Could you check a few things on this model? Use its own coordinates, in mm. A direction names the side the tool comes from. Give positions to 0.01 mm unless a question says otherwise; leave off trailing zeros. Loops run counter-clockwise (first coordinate to the right, second up) from the corner with the lowest first, then second, coordinate; pieces in that order, holes last. Notation, with made-up numbers: (83, 84) - (107, 84) arc R17 cw to (107, 101) - close; hole circle Ø8 at (3, -32). An arc over 180 degrees is marked (long way). Write each question's results on one line, items separated by ' | '. Start each with the question number.
(1) For pin 1 (2.5 mm diameter, centred on y = 28, z = 16.5, fed in from +X); pin 2 (2.5 mm diameter, centred on x = -2, z = 7, fed in from -Y); pin 3 (2 mm diameter, centred on x = -20.5, z = 11, fed in from +Y), each with a flat end and sliding along its axis, tell me the tip position at first contact or that it passes through.
(2) Suppose I cut it at C-C (z = 7.75). Please give me the cut outline in (x, y), and give its area (3 significant figures).
(3) I need wall thicknesses on line 1 (X direction, y = 35, z = 16); line 2 (Y direction, x = 0, z = 15.9); line 3 (Y direction, x = 0, z = 4.65). Which ranges of each line are inside material? Lowest first, please.
(4) Suppose I cut it at B-B (x = -10). Please give me the cut outline in (y, z).
(5) Suppose I cut it at D-D (x = 14.5). Please give me the cut outline in (y, z).
(6) If we mould it in two halves opening along X, with no side actions, what happens to faces 5 (the face through (8.894, 43.96, 10.902)), 6 (the face through (22.88, 44.49, 11.1)), 7 (the face through (0, 41, 18))? For each: released by +X, released by -X, zero draft, split by the parting line, or undercut.
(7) On a 3-axis mill with a long thin cutter (end or side, diameter ignored), from which of +Z, -Z, +X, -X, +Y, -Y can I reach the whole of each face in a straight line? I mean faces 1 (the face through (0.46, 28.84, 4.49)), 2 (the face through (-19, 31, 16)), 3 (the face through (2.211, 32.947, 16.479)), 4 (the face through (6, 22, 9)). Say none if no direction works.
(8) Suppose I cut it at A-A (x = 0). Please give me the cut outline in (y, z), and give its area (3 significant figures).
from build123d import *
from build123d.topology import SkipClean

# Parameters (mm, degrees)
CROQUIS3_W                   = 38
CROQUIS3_H                   = 38
SALIENTE_EXTRUIR9_DEPTH      = 1
SALIENTE_EXTRUIR10_START     = -11
SALIENTE_EXTRUIR10_OUTLINE_W = 38
SALIENTE_EXTRUIR10_OUTLINE_H = 38
SALIENTE_EXTRUIR10_DEPTH     = 10
CROQUIS13_W                  = 38
CROQUIS13_H                  = 38
SALIENTE_EXTRUIR15_DEPTH     = 3
CROQUIS14_R                  = 1.5
CORTAR_EXTRUIR1_DEPTH        = 14
CROQUIS15_W                  = 38
CROQUIS15_H                  = 24.129942315
CROQUIS15_R                  = 1.5
CROQUIS15_R_2                = 3.5
SALIENTE_EXTRUIR16_DEPTH     = 1
CORTAR_EXTRUIR2_DEPTH        = 14
CROQUIS17_R                  = 1.5
SALIENTE_EXTRUIR17_DEPTH     = 5
CROQUIS18_R                  = 1.5
CROQUIS18_W                  = 12
CROQUIS18_H                  = 12
SALIENTE_EXTRUIR18_DEPTH     = 5
CORTAR_EXTRUIR3_DEPTH        = 3
CROQUIS20_R                  = 3
CROQUIS20_R_2                = 1.5
SALIENTE_EXTRUIR19_DEPTH     = 3
REDONDEO11_R                 = 1


# Read off the part's stored shape, not the designer's step: Saliente-Extruir10
with BuildPart() as part:
    # Croquis3 → Saliente-Extruir9 (new body)
    with BuildSketch(Plane.XY.offset(5)):
        Polygon((19, -5.370057685), (26.870057685, 2.5), (26.870057685, 40.5), (19, 48.370057685), (-19, 48.370057685), (-26.870057685, 40.5), (-26.870057685, 2.5), (-19, -5.370057685), align=None)
        with Locations((0, 21.5)):
            Rectangle(CROQUIS3_W, CROQUIS3_H, mode=Mode.SUBTRACT)
    extrude(amount=-SALIENTE_EXTRUIR9_DEPTH)

    # Saliente-Extruir10 outline → Saliente-Extruir10 (add)
    with BuildSketch(Plane(origin=(0, 0, 4), x_dir=(-1, 0, 0), z_dir=(0, 0, -1)).offset(SALIENTE_EXTRUIR10_START)):
        Polygon((-26.870057685, 2.5), (-19, -5.370057685), (19, -5.370057685), (26.870057685, 2.5), (26.870057685, 40.5), (19, 48.370057685), (-19, 48.370057685), (-26.870057685, 40.5), align=None)
        with Locations((0, 21.5)):
            Rectangle(SALIENTE_EXTRUIR10_OUTLINE_W, SALIENTE_EXTRUIR10_OUTLINE_H, mode=Mode.SUBTRACT)
    extrude(amount=SALIENTE_EXTRUIR10_DEPTH)

    # Croquis13 → Saliente-Extruir15 (add)
    with BuildSketch(Plane.XY.offset(15)):
        with BuildLine():
            Line((-22.5, 44.870057685), (-22.5, -1))
            Line((-22.5, -1), (22.5, -1))
            Line((22.5, -1), (22.5, 44.870057685))
            Line((22.5, 44.870057685), (19.292893219, 48.077164466))
            ThreePointArc((19.292893219, 48.077164466), (18.96846987, 48.293937218), (18.585786438, 48.370057685))
            Line((18.585786438, 48.370057685), (-18.585786438, 48.370057685))
            ThreePointArc((-18.585786438, 48.370057685), (-18.96846987, 48.293937218), (-19.292893219, 48.077164466))
            Line((-19.292893219, 48.077164466), (-22.5, 44.870057685))
        make_face()
        with Locations((0, 21.5)):
            Rectangle(CROQUIS13_W, CROQUIS13_H, mode=Mode.SUBTRACT)
    extrude(amount=SALIENTE_EXTRUIR15_DEPTH)

    # Croquis14 → Cortar-Extruir1 (cut)
    with BuildSketch(Plane(origin=(0, 0, 4), x_dir=(-1, 0, 0), z_dir=(0, 0, -1))):
        with Locations((10, 44.97415474)):
            Circle(CROQUIS14_R)
        with Locations(Location((-10, 44.97415474, 0), (0, 0, 180))):
            Circle(CROQUIS14_R)
    extrude(amount=-CORTAR_EXTRUIR1_DEPTH, mode=Mode.SUBTRACT)

    # Croquis15 → Saliente-Extruir16 (add)
    with BuildSketch(Plane(origin=(0, 0, 4), x_dir=(-1, 0, 0), z_dir=(0, 0, -1))):
        with Locations((0, 28.435028843)):
            Rectangle(CROQUIS15_W, CROQUIS15_H)
        with Locations((0, 34.97415474)):
            Circle(CROQUIS15_R, mode=Mode.SUBTRACT)
        with Locations((0, 25.370057685)):
            Circle(CROQUIS15_R_2, mode=Mode.SUBTRACT)
    extrude(amount=-SALIENTE_EXTRUIR16_DEPTH)

    # Croquis16 → Cortar-Extruir2 (cut)
    with BuildSketch(Plane(origin=(0, 0, 4), x_dir=(-1, 0, 0), z_dir=(0, 0, -1))):
        Polygon((-19, 2.5), (-19, 16.370057685), (-26.870057685, 24.24011537), (-26.870057685, 2.5), (-19, -5.370057685), (19, -5.370057685), (26.870057685, 2.5), (26.870057685, 24.24011537), (19, 16.370057685), (19, 2.5), align=None)
    extrude(amount=-CORTAR_EXTRUIR2_DEPTH, mode=Mode.SUBTRACT)

    # Croquis17 → Saliente-Extruir17 (add)
    with SkipClean():  # the faces are left unmerged after this step: merging them gives an invalid solid
        with BuildSketch(Plane.XY.offset(5)):
            Polygon((6, 31.370057685), (6, 25.370057685), (6, 19.370057685), (6, 16.370057685), (19, 16.370057685), (19, 40.5), (-19, 40.5), (-19, 16.370057685), (-6, 16.370057685), (-6, 19.370057685), (-6, 31.370057685), align=None)
            with Locations((0, 34.97415474)):
                Circle(CROQUIS17_R, mode=Mode.SUBTRACT)
        extrude(amount=SALIENTE_EXTRUIR17_DEPTH)
    add(part.part.scale(1), mode=Mode.REPLACE)  # the faces are merged on a copy

    # Croquis18 → Saliente-Extruir18 (add)
    # profile 1 of 2: a face of its own
    with BuildSketch(Plane.XY.offset(10)):
        Polygon((-6, 31.370057685), (6, 31.370057685), (6, 16.370057685), (19, 16.370057685), (19, 40.5), (-19, 40.5), (-19, 16.370057685), (-6, 16.370057685), align=None)
        with Locations(Location((0, 34.97415474, 0), (0, 0, 180))):
            Circle(CROQUIS18_R, mode=Mode.SUBTRACT)
    # profile 2 of 2: a face of its own
    with BuildSketch(Plane.XY.offset(10)):
        with Locations((0, 25.370057685)):
            Rectangle(CROQUIS18_W, CROQUIS18_H)
    extrude(amount=SALIENTE_EXTRUIR18_DEPTH)

    # Croquis19 → Cortar-Extruir3 (cut)
    with BuildSketch(Plane.XY.offset(18)):
        Polygon((-22.5, 19.870057685), (-19, 16.370057685), (-19, 21.370057685), (-22.5, 21.370057685), align=None)
        Polygon((19, 16.370057685), (22.5, 19.870057685), (22.5, 21.370057685), (19, 21.370057685), align=None)
    extrude(amount=-CORTAR_EXTRUIR3_DEPTH, mode=Mode.SUBTRACT)

    # Croquis20 → Saliente-Extruir19 (add)
    with BuildSketch(Plane.XY.offset(15)):
        with Locations(Location((0, 34.97415474, 0), (0, 0, 180))):
            Circle(CROQUIS20_R)
        with Locations(Location((0, 34.97415474, 0), (0, 0, 180))):
            Circle(CROQUIS20_R_2, mode=Mode.SUBTRACT)
    extrude(amount=SALIENTE_EXTRUIR19_DEPTH)

    # Redondeo11
    redondeo11_edges = [part.edges().sort_by_distance(p)[0] for p in [
        (26.870057685, 40.5, 10),
        (19, 48.370057685, 10),
        (-19, 48.370057685, 10),
        (-26.870057685, 40.5, 10),
        (26.870057685, 24.24011537, 9.5),
        (19, 16.370057685, 9.5),
        (-26.870057685, 24.24011537, 9.5),
        (-19, 16.370057685, 9.5),
    ]]
    fillet(redondeo11_edges, radius=REDONDEO11_R)


solid = part.part
Output values:
1) pin 1: x = 22.5 | pin 2: y = 31.37 | pin 3: y = 47.87
2) outline: (-26.87, 24.65) arc R1 ccw to (-26.58, 23.95) - (-19.29, 16.66) arc R1 ccw to (-18.59, 16.37) - (-6, 16.37) - (-6, 31.37) - (6, 31.37) - (6, 16.37) - (18.59, 16.37) arc R1 ccw to (19.29, 16.66) - (26.58, 23.95) arc R1 ccw to (26.87, 24.65) - (26.87, 40.09) arc R1 ccw to (26.58, 40.79) - (19.29, 48.08) arc R1 ccw to (18.59, 48.37) - (-18.59, 48.37) arc R1 ccw to (-19.29, 48.08) - (-26.58, 40.79) arc R1 ccw to (-26.87, 40.09) - close; hole circle Ø3 at (-10, 44.97); hole circle Ø3 at (0, 34.97); hole circle Ø3 at (10, 44.97) | area: 1,390 mm2
3) line 1: -22.5 to -19, -3 to -1.5, 1.5 to 3, 19 to 22.5 | line 2: 31.97 to 33.47, 36.47 to 37.97, 40.5 to 48.37 | line 3: 16.37 to 21.87, 28.87 to 33.47, 36.47 to 48.37
4) outline: (16.37, 4) - (43.47, 4) - (43.47, 18) - (40.5, 18) - (40.5, 15) - (16.37, 15) - close; (46.47, 4) - (48.37, 4) - (48.37, 18) - (46.47, 18) - close
5) outline: (16.37, 4) - (48.37, 4) - (48.37, 18) - (40.5, 18) - (40.5, 15) - (16.37, 15) - close
6) face 5: undercut | face 6: released by +X | face 7: zero draft
7) face 1: -Z | face 2: +Z, -Y | face 3: +Z | face 4: -Y
8) outline: (16.37, 4) - (21.87, 4) - (21.87, 5) - (16.37, 5) - close; (19.37, 10) - (31.37, 10) - (31.37, 5) - (28.87, 5) - (28.87, 4) - (33.47, 4) - (33.47, 18) - (31.97, 18) - (31.97, 15) - (19.37, 15) - close; (36.47, 4) - (48.37, 4) - (48.37, 18) - (40.5, 18) - (40.5, 15) - (37.97, 15) - (37.97, 18) - (36.47, 18) - close | area: 255 mm2
